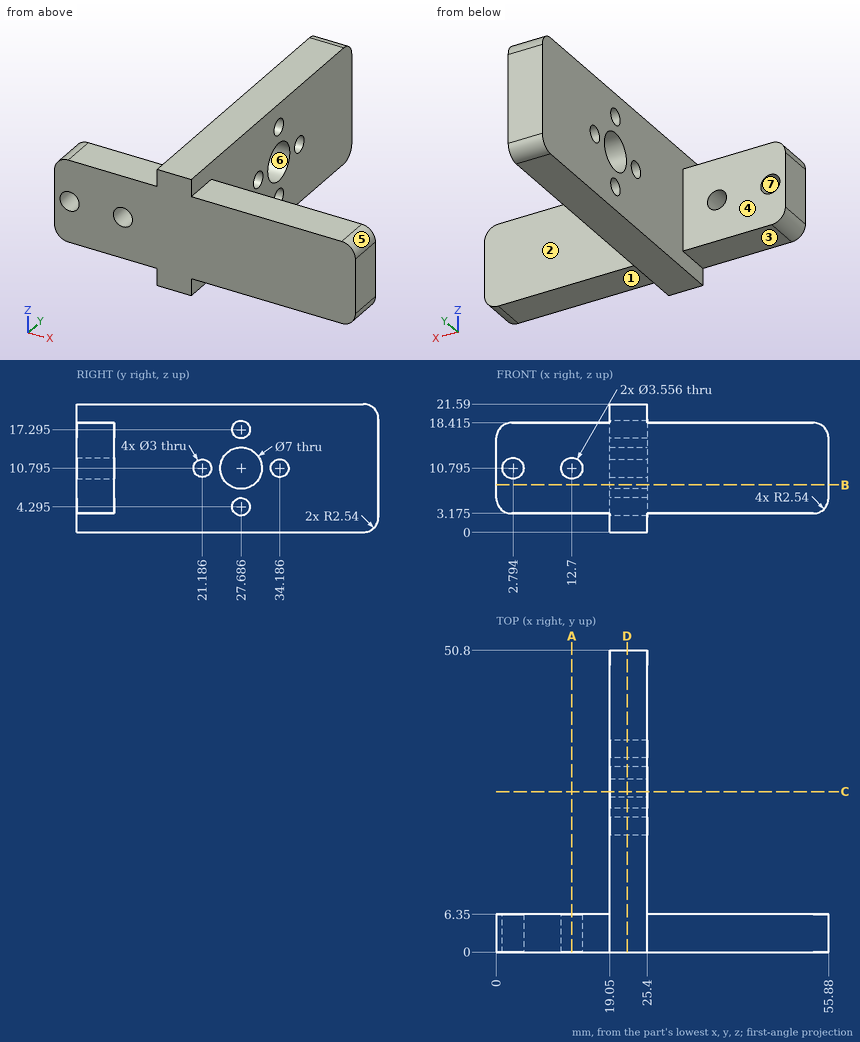
Geometry: see drawing. Coordinates: mm, zero at the bounding-box minimum. A direction names the side the tool comes from. Give positions to 0.01 mm unless a question says otherwise; leave off trailing zeros. Write each loop counter-clockwise with the first axis right and the second up, starting at its lowest first coordinate (ties: lowest second). Pieces come first, ordered by that corner, then holes. Notation, with made-up numbers: (9.5, -17) -> (51.5, -17) arc R20 cw to (51.5, 1) -> close; hole circle Ø10 at (13, 80.5). An arc over 180 degrees is marked (long way). Use one line per item in the form item = value. Start each with the question number.
1) Draft query along X for the marked faces 5, 6 and 7. Return one class per face: pulls with the +X half, pulls with the -X half, needs draft (parallel to the pull), parting line crosses it, or undercut.
2) Section query A-A on x = 12.7. Return the cut outline in (y, z) (3 decimals).
3) Section query B-B on z = 8. Return the cut outline in (x, y), then the cut area to 3 significant figures.
4) Set-up query: the marked faces 1, 2, 3 and 4. Return all of +Z, -Z, +X, -X, +Y, -Y with unobstructed straight access to the full face (end or side cutting, diameter ignored); none if empty.
5) Section query D-D on x = 22. Return the cut outline in (y, z) (3 decimals), then the cut area to 3 significant figures.
6) Ray query, probe 1 along Z at (x, y) = (12.7, 2.5) (3 decimals); probe 2 along Y at (x, z) = (3, 3.5); probe 3 along X at (y, z) = (14.5, 11). Return the intervals inside material, ascending. Write a range as from..to.
7) Section query C-C on y = 27. Return the cut outline in (x, z).
8) Pin query (flat end, axial travel): pin 1 (4 mm diameter, centred on x = 12.7, z = 10.795, fed in from +Y); pin 2 (1.8 mm diameter, centred on y = 27.686, z = 17.295, fed in from +X); pin 3 (8 mm diameter, centred on y = 40.5, z = 9, fed in from -X); pin 4 (3 mm diameter, centred on x = 36.5, y = 3, fed in from +Z) (3 decimals). Return the tip coordinate at first contact, or that it passes through.
Outcome:
q1.face_5 = pulls with the +X half
q1.face_6 = needs draft
q1.face_7 = undercut
q2.outline = (0, 3.175) -> (6.35, 3.175) -> (6.35, 9.017) -> (0, 9.017) -> close; (0, 12.573) -> (6.35, 12.573) -> (6.35, 18.415) -> (0, 18.415) -> close
q3.outline = (0, 0) -> (55.88, 0) -> (55.88, 6.35) -> (25.4, 6.35) -> (25.4, 25.58) -> (19.05, 25.58) -> (19.05, 6.35) -> (0, 6.35) -> close; (19.05, 29.79) -> (25.4, 29.79) -> (25.4, 50.8) -> (19.05, 50.8) -> close
q3.area = 610 mm^2
q4.face_1 = -Z, +X, +Y, -Y
q4.face_2 = +Z, -Z, +X, +Y
q4.face_3 = -Z, -X, +Y, -Y
q4.face_4 = +Z, -Z, -X, +Y
q5.outline = (0, 0) -> (48.26, 0) arc R2.54 ccw to (50.8, 2.54) -> (50.8, 19.05) arc R2.54 ccw to (48.26, 21.59) -> (0, 21.59) -> close; hole circle Ø3 at (21.186, 10.795); hole circle Ø7 at (27.686, 10.795); hole circle Ø3 at (27.686, 4.295); hole circle Ø3 at (27.686, 17.295); hole circle Ø3 at (34.186, 10.795)
q5.area = 1,030 mm^2
q6.probe_1 = 3.175..9.017, 12.573..18.415
q6.probe_2 = 0..6.35
q6.probe_3 = 19.05..25.4
q7.outline = (19.05, 0) -> (25.4, 0) -> (25.4, 2.96) -> (19.05, 2.96) -> close; (19.05, 5.63) -> (25.4, 5.63) -> (25.4, 7.36) -> (19.05, 7.36) -> close; (19.05, 14.23) -> (25.4, 14.23) -> (25.4, 15.96) -> (19.05, 15.96) -> close; (19.05, 18.63) -> (25.4, 18.63) -> (25.4, 21.59) -> (19.05, 21.59) -> close
q8.pin_1 = 6.35
q8.pin_2 = through
q8.pin_3 = 19.05
q8.pin_4 = 18.415
